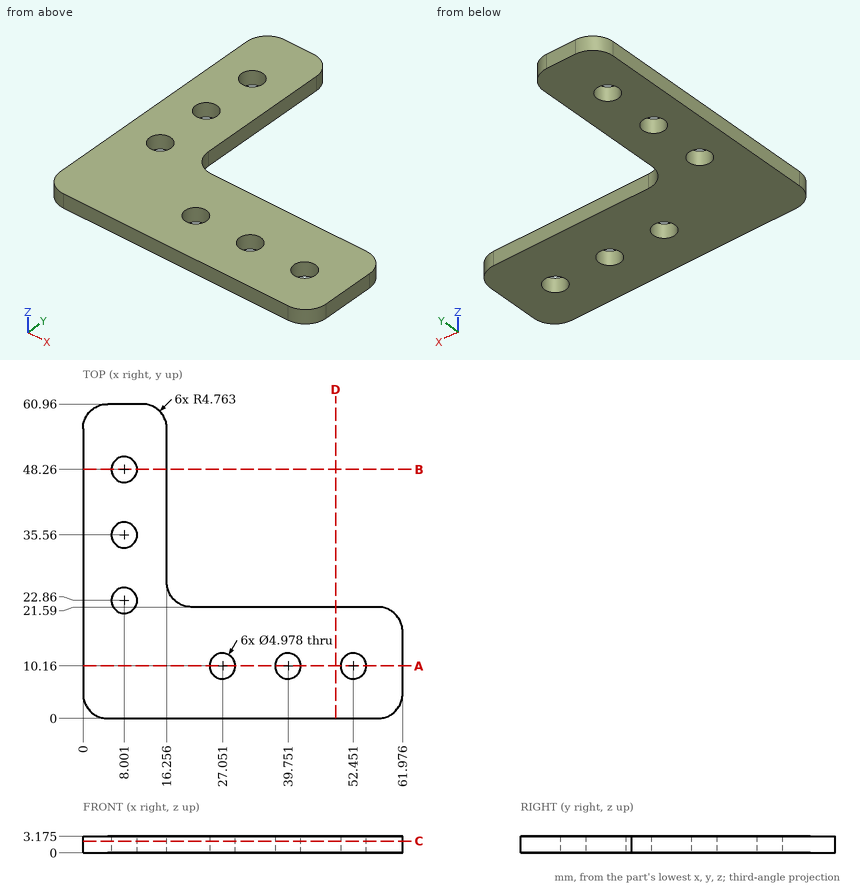
Design review of the part shown in the three views and the two pictorial views. Dimensions are in mm from the part's minimum x, y and z. Give positions to 0.01 mm unless a question says otherwise; leave off trailing zeros. Loops run counter-clockwise (first coordinate to the right, second up) from the corner with the lowest first, then second, coordinate; pieces in that order, holes last. Notation, with made-up numbers: M -11.75,30.5 L 33.25,30.5 A13 ccw 33.25,47.5 Z; hole C -0.75,15 d5. An arc over 180 degrees is marked long. Put each result on its own line as item: value. Start each with the question number.
(1) Add section B-B, the plane y = 48.26. Write out the cut boundary in (x, z) (1 decimal).
(2) Wall thickness on L1, parallel to Y at x = 8.5, z = 2.4; L2, parallel to X at y = 48.5, z = 0.95 (1 decimal); L3, parallel to X at y = 17, z = 1.5: over which ranges is each line inside the solid? List them lowest first.
(3) Add section D-D, the plane x = 49. Write out the cut boundary in (y, z) (1 decimal).
(4) Add section C-C, the plane z = 2.25. Give the number of separate pieces and of enclosed holes in the cut face, then the cut area to 3 significant figures.
(5) Add section A-A, the plane y = 10.16. Write out the cut boundary in (x, z) (1 decimal), then the cut area to 3 significant figures.
(6) For pin 1 (4.5 mm diameter, centred on x = 8.001, y = 35.56, fed in from -Z); pin 2 (1 mm diameter, centred on y = 40.5, z = 2, fed in from +X), all flat-tipped, find the tip position at first contact; note any pin that passes through.
Result:
1. outline: M 0,0 L 5.5,0 L 5.5,3.2 L 0,3.2 Z; M 10.5,0 L 16.3,0 L 16.3,3.2 L 10.5,3.2 Z
2. L1: y = 0 to 20.42, 25.3 to 33.12, 38 to 45.82, 50.7 to 60.96
2. L2: x = 0 to 5.5, 10.5 to 16.3
2. L3: x = 0 to 61.97
3. outline: M 0,0 L 21.6,0 L 21.6,3.2 L 0,3.2 Z
4. separate pieces: 1
4. enclosed holes: 6
4. area: 1,840 mm^2
5. outline: M 0,0 L 24.6,0 L 24.6,3.2 L 0,3.2 Z; M 29.5,0 L 37.3,0 L 37.3,3.2 L 29.5,3.2 Z; M 42.2,0 L 50,0 L 50,3.2 L 42.2,3.2 Z; M 54.9,0 L 62,0 L 62,3.2 L 54.9,3.2 Z
5. area: 149 mm^2
6. pin 1: passes through
6. pin 2: stops at x = 16.26
